```python
from build123d import *

# Parameters (mm, degrees)
SKETCH1_R         = 15.875
EXTRUDE1_DEPTH    = 3.175
EXTRUDE2_DEPTH    = 3.175
SKETCH3_R         = 1.5875
EXTRUDE3_DEPTH    = 83.249530363
CIRPATTERN1_COUNT = 8
SKETCH4_R         = 1.5875
EXTRUDE4_DEPTH    = 78.738955692
CIRPATTERN2_COUNT = 4


with BuildPart() as part:
    # Sketch1 → Extrude1 (new body)
    with BuildSketch(Plane.XY):
        with BuildLine():
            Line((-12.7, 25.597668351), (-12.7, 44.45))
            Line((-12.7, 44.45), (12.7, 44.45))
            Line((12.7, 44.45), (12.7, 25.597668351))
            ThreePointArc((12.7, 25.597668351), (0, -28.575), (-12.7, 25.597668351))
        make_face()
        Circle(SKETCH1_R, mode=Mode.SUBTRACT)
    extrude(amount=EXTRUDE1_DEPTH)

    # Sketch2 → Extrude2 (add)
    with BuildSketch(Plane(origin=(0, 23.8125, 23.8125), x_dir=(-1, 0, 0), z_dir=(0, 0.7071067811865488, 0.7071067811865462))):
        with BuildLine():
            Line((12.7, -29.185832393), (12.7, -54.585832393))
            ThreePointArc((12.7, -54.585832393), (0, -67.285832393), (-12.7, -54.585832393))
            Line((-12.7, -54.585832393), (-12.7, -29.185832393))
            Line((-12.7, -29.185832393), (12.7, -29.185832393))
        make_face()
    extrude(amount=-EXTRUDE2_DEPTH)

    # Sketch3 → Extrude3 (cut, through all)
    with BuildSketch(Plane.XY.offset(3.175)):
        with Locations((0, 22.225)):
            Circle(SKETCH3_R)
    extrude3 = extrude(amount=-EXTRUDE3_DEPTH, mode=Mode.SUBTRACT)

    # CirPattern1: Extrude3 ×8 about axis
    cirpattern1_axis = Axis((0, 0, 0), (0, 0, 1))
    for i in range(1, CIRPATTERN1_COUNT):
        add(extrude3.rotate(cirpattern1_axis, i * 360 / CIRPATTERN1_COUNT), mode=Mode.SUBTRACT)

    # Sketch4 → Extrude4 (cut, through all)
    with BuildSketch(Plane(origin=(0, 23.8125, 23.8125), x_dir=(1, 0, 0), z_dir=(0, 0.7071067811865488, 0.7071067811865462))):
        with Locations(Location((0, 60.935832393, 0), (0, 0, 270))):
            Circle(SKETCH4_R)
    extrude4 = extrude(amount=-EXTRUDE4_DEPTH, mode=Mode.SUBTRACT)

    # CirPattern2: Extrude4 ×4 about axis
    cirpattern2_axis = Axis((0, 38.598012242, -38.598012242), (0, 0.7071067811865488, 0.7071067811865462))
    for i in range(1, CIRPATTERN2_COUNT):
        add(extrude4.rotate(cirpattern2_axis, i * 360 / CIRPATTERN2_COUNT), mode=Mode.SUBTRACT)


solid = part.part
```
Model file for the job. Use its own axes, mm. A direction names the side the tool comes from. Round coordinates to 2 decimals unless told otherwise and drop trailing zeros. Order: outer loops, then holes, each group sorted by start corner. A loop starts at its lowest first (then second) coordinate and runs counter-clockwise, first axis right, second up. Notation, with made-up numbers: (81, -37) -> (137, -37) arc R20 ccw to (137, -10) -> close; hole circle Ø9 at (-10.5, 14). An arc over 180 degrees is marked (long way). Use one line per item in the form item = value.
Item 1: Cut at D-D, the plane x = 11. Write the cut outline in (y, z) (3 decimals).
Returned:
outline = (-26.373, 0) -> (-11.446, 0) -> (-11.446, 3.175) -> (-26.373, 3.175) -> close; (11.446, 0) -> (43.135, 0) -> (64.654, -21.519) -> (66.899, -19.274) -> (44.45, 3.175) -> (11.446, 3.175) -> close
Item 2: Cut at A-A, the plane y = 0. Write the cut outline in (x, z) (1 decimal).
Returned:
outline = (-28.6, 0) -> (-23.8, 0) -> (-23.8, 3.2) -> (-28.6, 3.2) -> close; (-20.6, 0) -> (-15.9, 0) -> (-15.9, 3.2) -> (-20.6, 3.2) -> close; (15.9, 0) -> (20.6, 0) -> (20.6, 3.2) -> (15.9, 3.2) -> close; (23.8, 0) -> (28.6, 0) -> (28.6, 3.2) -> (23.8, 3.2) -> close
Item 3: Flat gauge pins, fed straight in: pin 1 Ø3.5 at (x, y) = (-22.225, 0) entering from -Z; pin 2 Ø6 at (y, z) = (45, -2.5) entering from +X; pin 3 Ø1.5 at (y, z) = (-9.5, -0.5) entering from -X. Where does each tip first touch, or does it go through?
Returned:
pin_1 = 0
pin_2 = 12.7
pin_3 = -27.14
Item 4: Cut at B-B, the plane z = 1. Give the number of separate pieces and of enclosed holes in the cut face, and give its area (3 significant figures).
Returned:
separate_pieces = 1
enclosed_holes = 9
area = 2,190 mm^2
Item 5: Pull direction Z, two halves, no side cores. Call faces 4 (the face through (4.836, 60.967, -15.555)), 5 (the face through (-6, 16, 0)), 6 (the face through (0, 17, 3.175)), 7 (the face through (-14.2, 15.24, 1.61)): released by +Z, released by -Z, zero draft, split by the parting line, or undercut.
Returned:
face_4 = undercut
face_5 = released by -Z
face_6 = released by +Z
face_7 = zero draft
Item 6: Tool access for faces 1 (the face through (-12.7, 47, -3)), 2 (the face through (12.7, 46, -2)), 3 (the face through (0.477, 64.723, -19.312)): list every direction of +Z, -Z, +X, -X, +Y, -Y with a clear straight run to the whole face (end or side of a thin tool).
Returned:
face_1 = +Z, -Z, -X, +Y
face_2 = +Z, -Z, +X, +Y
face_3 = none
Item 7: Drill centre lines: line 1 (Z direction, x = 22.5, y = -12.5) (3 decimals); line 2 (X direction, y = 26.5, z = 1.5); line 3 (X direction, y = -4, z = 1.5). Where is each one in solid material? Low to high.
Returned:
line_1 = 0 to 3.175
line_2 = -12.7 to 12.7
line_3 = -28.29 to -15.36, 15.36 to 28.29
